Geometry check sheet. Reference: the model listing, model coordinates, mm. A direction names the side the tool comes from. Give positions to 0.01 mm unless a question says otherwise; leave off trailing zeros. Write each loop counter-clockwise with the first axis right and the second up, starting at its lowest first coordinate (ties: lowest second). Pieces come first, ordered by that corner, then holes. Notation, with made-up numbers: M -30,44 L 15,44 A23 ccw 15,81 Z; hole C 83,-28.5 d5. An arc over 180 degrees is marked long. Write each question's results on one line, items separated by ' | '.
```python
from build123d import *

# Parameters (mm, degrees)
F0_R          = 4.675
F0_R_2        = 3.175
F1_DEPTH      = 15
F1_DEPTH_BACK = 2.5
F2_R          = 6
F2_R_2        = 4.5
F3_DEPTH      = 15
F3_DEPTH_BACK = 2.5


with BuildPart() as f1:
    # F0 (on Front) → F1 (new body, two sides)
    with BuildSketch(Plane.XZ) as f1_sk:
        Circle(F0_R)
        Circle(F0_R_2, mode=Mode.SUBTRACT)
    extrude(amount=F1_DEPTH)
    extrude(f1_sk.sketch, amount=-F1_DEPTH_BACK)

    # F2 (on Front) → F3 (join, two sides)
    with BuildSketch(Plane.XZ) as f3_sk:
        Circle(F2_R)
        Circle(F2_R_2, mode=Mode.SUBTRACT)
    extrude(amount=-F3_DEPTH)
    extrude(f3_sk.sketch, amount=F3_DEPTH_BACK)


solid = f1.part
```
Q1. Section check D-D (x = -3.75). Enter the section's corners in (y, z), then the cut area to 3 significant figures.
Answer key:
outline: M -15,-2.79 L -2.5,-2.79 L -2.5,-4.68 L 15,-4.68 L 15,-2.49 L 2.5,-2.49 L 2.5,2.49 L 15,2.49 L 15,4.68 L -2.5,4.68 L -2.5,2.79 L -15,2.79 Z | area: 172 mm2
Q2. Release check for a two-part mould opening along Z. For faces 1 (the face through (2, 2.5, -3)), 2 (the face through (3, -2.5, -4)), 3 (the face through (-1.013, -8.838, -4.564)) record: released by +Z, released by -Z, zero draft, split by the parting line, or undercut.
Answer key:
face 1: undercut | face 2: zero draft | face 3: split by the parting line
Q3. Depth check by flat-ended pin: P1, Ø6, axis at x = 0, z = 0.5, coming from the +Y side; P2, Ø2, axis at y = -10.5, z = -2, coming from the -X side; P3, Ø1.5, axis at y = -11.5, z = 0.5, coming from the +X side (3 decimals). Enter the tip coordinate at first touch or a pass-through.
Answer key:
P1: stops at y = 2.5 | P2: stops at x = -4.57 | P3: stops at x = 4.675
Q4. Section check C-C (y = -13). Enter the section's corners in (x, z) (3 decimals), then the cut area to 3 significant figures.
Answer key:
outline: C 0,0 d9.35; hole C 0,0 d6.35 | area: 37.0 mm2
Q5. Access from +Z, -Z, +X, -X, +Y, -Y to the whole of each face (thin tool, end or side, straight path). Record for faces 4 (the face through (-1.4, 15, 4.5)), 5 (the face through (-0.59, 8.66, 4.46)).
Answer key:
face 4: +Z, -Z, +X, -X, +Y | face 5: +Y
Q6. Material ranges on probe 1 along Z at (x, y) = (0.25, 5.25); probe 2 along Z at (x, y) = (0, -10) (3 decimals); probe 3 along Y at (x, z) = (2.25, -2.75), recorded low to high. Write a range as [from, to].
Answer key:
probe 1: z = [-5.99, -4.49], [4.49, 5.99] | probe 2: z = [-4.675, -3.175], [3.175, 4.675] | probe 3: y = [-15, 2.5]
Q7. Section check A-A (x = 0). Enter the section's corners in (y, z) (3 decimals), then the cut area to 3 significant figures.
Answer key:
outline: M -15,-4.675 L -2.5,-4.675 L -2.5,-6 L 15,-6 L 15,-4.5 L 2.5,-4.5 L 2.5,-3.175 L -15,-3.175 Z; M -15,3.175 L 2.5,3.175 L 2.5,4.5 L 15,4.5 L 15,6 L -2.5,6 L -2.5,4.675 L -15,4.675 Z | area: 103 mm2
Q8. Section check B-B (z = -2.25). Enter the section's corners in (x, y), then the cut area to 3 significant figures.
Answer key:
outline: M -5.56,-2.5 L -4.1,-2.5 L -4.1,-15 L -2.24,-15 L -2.24,2.5 L -3.9,2.5 L -3.9,15 L -5.56,15 Z; M 2.24,-15 L 4.1,-15 L 4.1,-2.5 L 5.56,-2.5 L 5.56,15 L 3.9,15 L 3.9,2.5 L 2.24,2.5 Z | area: 121 mm2
